from build123d import *

# Parameters (mm, degrees)
SKETCH1_W           = 130
SKETCH1_H           = 45
BOSS_EXTRUDE1_DEPTH = 10
SKETCH2_W           = 110
SKETCH2_H           = 12
CUT_EXTRUDE1_DEPTH  = 7.8
SKETCH4_R           = 2
CUT_EXTRUDE3_DEPTH  = 11
SKETCH5_R           = 4
CUT_EXTRUDE4_DEPTH  = 3
SKETCH6_W           = 41
SKETCH6_H           = 41
CUT_EXTRUDE5_DEPTH  = 7.8


with BuildPart() as part:
    # Sketch1 → Boss-Extrude1 (new body)
    with BuildSketch(Plane.XY):
        with Locations((65, 22.5)):
            Rectangle(SKETCH1_W, SKETCH1_H)
    extrude(amount=BOSS_EXTRUDE1_DEPTH)

    # Sketch2 → Cut-Extrude1 (cut)
    with BuildSketch(Plane(origin=(0, 0, 0), x_dir=(-1, 0, 0), z_dir=(0, 0, -1))):
        with Locations((-75, 22.5)):
            Rectangle(SKETCH2_W, SKETCH2_H)
    extrude(amount=-CUT_EXTRUDE1_DEPTH, mode=Mode.SUBTRACT)

    # Sketch4 → Cut-Extrude3 (cut, through all)
    with BuildSketch(Plane.XY.offset(10)):
        with Locations((55, 37.5)):
            Circle(SKETCH4_R)
        with Locations((115, 37.5)):
            Circle(SKETCH4_R)
        with Locations((115, 7.5)):
            Circle(SKETCH4_R)
        with Locations((55, 7.5)):
            Circle(SKETCH4_R)
    extrude(amount=-CUT_EXTRUDE3_DEPTH, mode=Mode.SUBTRACT)

    # Sketch5 → Cut-Extrude4 (cut)
    with BuildSketch(Plane.XY.offset(10)):
        with Locations((55, 37.5)):
            Circle(SKETCH5_R)
        with Locations((115, 37.5)):
            Circle(SKETCH5_R)
        with Locations((115, 7.5)):
            Circle(SKETCH5_R)
        with Locations((55, 7.5)):
            Circle(SKETCH5_R)
    extrude(amount=-CUT_EXTRUDE4_DEPTH, mode=Mode.SUBTRACT)

    # Sketch6 → Cut-Extrude5 (cut)
    with BuildSketch(Plane(origin=(0, 0, 0), x_dir=(-1, 0, 0), z_dir=(0, 0, -1))):
        with Locations((-27, 22.5)):
            Rectangle(SKETCH6_W, SKETCH6_H)
    extrude(amount=-CUT_EXTRUDE5_DEPTH, mode=Mode.SUBTRACT)


solid = part.part
For this review, take the finished solid that the model builds, in its own axes (mm). A direction names the side the tool comes from. Coordinates: 2 decimals unless noted, no trailing zeros. Order: outer loops, then holes, each group sorted by start corner. A loop starts at its lowest first (then second) coordinate and runs counter-clockwise, first axis right, second up. Notation, with made-up numbers: (-9, 13) - (6, 13) arc R22 cw to (6, 23) - close; hole circle Ø3 at (71, 64.5). An arc over 180 degrees is marked (long way). Answer as CSV lines item,"result". Start each with the question number.
1) Add section A-A (x = 55). State the section outline as (y, z) points, then the cut area to 3 significant figures.
2) Draft analysis for pull direction X (two halves, no side actions). For faces 4 (the flat face through (64, 0, 5)), 5 (the flat face through (0, 22, 5)), 6 (the flat face through (47.5, 36, 4)), state which applies: +X half, -X half, draft (parallel to the pull), parting line (faces both ways), or undercut.
3) Machinability: for faces 1 (the flat face through (117, 36, 7)), 2 (the flat face through (89, 16.5, 4)), 3 (the flat face through (55, 23, 7.8)), which of the approach directions +Z, -Z, +X, -X, +Y, -Y give a long, thin tool a straight path to every point of the face, cutting with its end or side? Answer none if there is none.
4) Add section B-B (y = 7.5). State the section outline as (x, z) points.
5) Insertion check: P1, Ø4, axis at y = 19, z = 3, coming from the +X side; P2, Ø2.5, axis at x = 55, y = 39, coming from the +Z side. Each pin has a flat end and moves straight along its axis. Give the tip position at first contact, or say it passes through.
6) Add section C-C (z = 1.75). State the section outline as (x, y) points.
7) To check wall thickness, follow line 1 along Y through (x, z) = (55, 9.45); line 2 along Y through (x, z) = (55, 4); line 3 along Y through (x, z) = (115, 7.6). State the ranges of each line that lie inside material, in increasing order. Write a range as [from, to].
8) Add section D-D (x = 89.5). State the section outline as (y, z) points.
Result:
1,outline,"(0, 0) - (5.5, 0) - (5.5, 7) - (3.5, 7) - (3.5, 10) - (0, 10) - close; (9.5, 0) - (16.5, 0) - (16.5, 7.8) - (28.5, 7.8) - (28.5, 0) - (35.5, 0) - (35.5, 7) - (33.5, 7) - (33.5, 10) - (11.5, 10) - (11.5, 7) - (9.5, 7) - close; (39.5, 0) - (45, 0) - (45, 10) - (41.5, 10) - (41.5, 7) - (39.5, 7) - close"
1,area,"252 mm^2"
2,face 4,"draft"
2,face 5,"-X half"
2,face 6,"undercut"
3,face 1,"+Z"
3,face 2,"-Z, +X"
3,face 3,"-Z"
4,outline,"(0, 0) - (6.5, 0) - (6.5, 7.8) - (47.5, 7.8) - (47.5, 0) - (53, 0) - (53, 7) - (51, 7) - (51, 10) - (0, 10) - close; (57, 0) - (113, 0) - (113, 7) - (111, 7) - (111, 10) - (59, 10) - (59, 7) - (57, 7) - close; (117, 0) - (130, 0) - (130, 10) - (119, 10) - (119, 7) - (117, 7) - close"
5,P1,"x = 6.5"
5,P2,"z = 7"
6,outline,"(0, 0) - (130, 0) - (130, 16.5) - (47.5, 16.5) - (47.5, 2) - (6.5, 2) - (6.5, 43) - (47.5, 43) - (47.5, 28.5) - (130, 28.5) - (130, 45) - (0, 45) - close; hole circle Ø4 at (55, 7.5); hole circle Ø4 at (55, 37.5); hole circle Ø4 at (115, 7.5); hole circle Ø4 at (115, 37.5)"
7,line 1,"[0, 3.5], [11.5, 33.5], [41.5, 45]"
7,line 2,"[0, 5.5], [9.5, 16.5], [28.5, 35.5], [39.5, 45]"
7,line 3,"[0, 3.5], [11.5, 16.5], [28.5, 33.5], [41.5, 45]"
8,outline,"(0, 0) - (16.5, 0) - (16.5, 7.8) - (28.5, 7.8) - (28.5, 0) - (45, 0) - (45, 10) - (0, 10) - close"
